from build123d import *

# Parameters (mm, degrees)
F1_DEPTH  = 93
F3_DEPTH  = 25
F4_W      = 3
F4_H      = 15.738895
F4_H_2    = 121.261105
F5_DEPTH  = 15
F6_DEPTH  = 15
F7_DEPTH  = 15
F8_DEPTH  = 15
F9_DEPTH  = 15
F10_DEPTH = 15
F11_DEPTH = 15
F4_H_3    = 121.394625
F12_DEPTH = 15
F13_DEPTH = 15
F14_DEPTH = 15
F15_DEPTH = 15
F16_DEPTH = 15
F17_DEPTH = 15
F18_DEPTH = 15
F19_DEPTH = 15
F20_W     = 23
F20_H     = 10
F21_DEPTH = 0.2
F22_R     = 2.5
F23_DEPTH = 2
F24_DEPTH = 2


with BuildPart() as f1:
    # F0 (on Front) → F1 (new body)
    with BuildSketch(Plane.XZ):
        with BuildLine():
            Line((191.195573, 236.532636), (-173.804427, 236.532636))
            ThreePointArc((-173.804427, 236.532636), (-184.411028, 232.139238), (-188.804427, 221.532636))
            Line((-188.804427, 221.532636), (-188.804427, -78.467364))
            ThreePointArc((-188.804427, -78.467364), (-184.411028, -89.073966), (-173.804427, -93.467364))
            Line((-173.804427, -93.467364), (191.195573, -93.467364))
            Line((191.195573, -93.467364), (191.195573, 236.532636))
        make_face()
        with BuildLine():
            ThreePointArc((-181.804427, 221.532636), (-179.461281, 227.18949), (-173.804427, 229.532636))
            Line((-173.804427, 229.532636), (184.195573, 229.532636))
            Line((184.195573, 229.532636), (184.195573, -86.467364))
            Line((184.195573, -86.467364), (-173.804427, -86.467364))
            ThreePointArc((-173.804427, -86.467364), (-179.461281, -84.124218), (-181.804427, -78.467364))
            Line((-181.804427, -78.467364), (-181.804427, 221.532636))
        make_face(mode=Mode.SUBTRACT)
    extrude(amount=F1_DEPTH)

    # F2 (on face) → F3 (cut)
    with BuildSketch(Plane.YZ.offset(191.195573)):
        Polygon((-6, 128.456), (-6, 226.532636), (-93, 226.532636), (-93, 68.456), (-48, 68.456), (-48, 128.456), align=None)
    extrude(amount=-F3_DEPTH, mode=Mode.SUBTRACT)

    # F4 (on face) → F5 (cut)
    with BuildSketch(Plane(origin=(-188.804427, 0, 0), x_dir=(0, -1, 0), z_dir=(-1, 0, 0))):
        with Locations((88.5, -86.336811)):
            Rectangle(F4_W, F4_H)
        with Locations((88.5, -17.836812)):
            Rectangle(F4_W, F4_H_2)
    extrude(amount=-F5_DEPTH, mode=Mode.SUBTRACT)

    # F4 (on face) → F6 (cut)
    with BuildSketch(Plane(origin=(-188.804427, 0, 0), x_dir=(0, -1, 0), z_dir=(-1, 0, 0))):
        with Locations((82.5, -17.836812)):
            Rectangle(F4_W, F4_H_2)
        with Locations((82.5, -86.336811)):
            Rectangle(F4_W, F4_H)
    extrude(amount=-F6_DEPTH, mode=Mode.SUBTRACT)

    # F4 (on face) → F7 (cut)
    with BuildSketch(Plane(origin=(-188.804427, 0, 0), x_dir=(0, -1, 0), z_dir=(-1, 0, 0))):
        with Locations((76.5, -17.836812)):
            Rectangle(F4_W, F4_H_2)
        with Locations((76.5, -86.336811)):
            Rectangle(F4_W, F4_H)
    extrude(amount=-F7_DEPTH, mode=Mode.SUBTRACT)

    # F4 (on face) → F8 (cut)
    with BuildSketch(Plane(origin=(-188.804427, 0, 0), x_dir=(0, -1, 0), z_dir=(-1, 0, 0))):
        with Locations((70.5, -17.836812)):
            Rectangle(F4_W, F4_H_2)
        with Locations((70.5, -86.336811)):
            Rectangle(F4_W, F4_H)
    extrude(amount=-F8_DEPTH, mode=Mode.SUBTRACT)

    # F4 (on face) → F9 (cut)
    with BuildSketch(Plane(origin=(-188.804427, 0, 0), x_dir=(0, -1, 0), z_dir=(-1, 0, 0))):
        with Locations((64.5, -17.836812)):
            Rectangle(F4_W, F4_H_2)
        with Locations((64.5, -86.336811)):
            Rectangle(F4_W, F4_H)
    extrude(amount=-F9_DEPTH, mode=Mode.SUBTRACT)

    # F4 (on face) → F10 (cut)
    with BuildSketch(Plane(origin=(-188.804427, 0, 0), x_dir=(0, -1, 0), z_dir=(-1, 0, 0))):
        with Locations((58.5, -86.336811)):
            Rectangle(F4_W, F4_H)
        with Locations((58.5, -17.836812)):
            Rectangle(F4_W, F4_H_2)
    extrude(amount=-F10_DEPTH, mode=Mode.SUBTRACT)

    # F4 (on face) → F11 (cut)
    with BuildSketch(Plane(origin=(-188.804427, 0, 0), x_dir=(0, -1, 0), z_dir=(-1, 0, 0))):
        with Locations((52.5, -17.836812)):
            Rectangle(F4_W, F4_H_2)
        with Locations((52.5, -86.336811)):
            Rectangle(F4_W, F4_H)
    extrude(amount=-F11_DEPTH, mode=Mode.SUBTRACT)

    # F4 (on face) → F12 (cut)
    with BuildSketch(Plane(origin=(-188.804427, 0, 0), x_dir=(0, -1, 0), z_dir=(-1, 0, 0))):
        with Locations((46.5, -86.336811)):
            Rectangle(F4_W, F4_H)
        with Locations((46.5, -17.770052)):
            Rectangle(F4_W, F4_H_3)
    extrude(amount=-F12_DEPTH, mode=Mode.SUBTRACT)

    # F4 (on face) → F13 (cut)
    with BuildSketch(Plane(origin=(-188.804427, 0, 0), x_dir=(0, -1, 0), z_dir=(-1, 0, 0))):
        with Locations((40.5, -17.770052)):
            Rectangle(F4_W, F4_H_3)
        with Locations((40.5, -86.336811)):
            Rectangle(F4_W, F4_H)
    extrude(amount=-F13_DEPTH, mode=Mode.SUBTRACT)

    # F4 (on face) → F14 (cut)
    with BuildSketch(Plane(origin=(-188.804427, 0, 0), x_dir=(0, -1, 0), z_dir=(-1, 0, 0))):
        with Locations((40.5, -17.770052)):
            Rectangle(F4_W, F4_H_3)
        with Locations((40.5, -86.336811)):
            Rectangle(F4_W, F4_H)
    extrude(amount=-F14_DEPTH, mode=Mode.SUBTRACT)

    # F4 (on face) → F15 (cut)
    with BuildSketch(Plane(origin=(-188.804427, 0, 0), x_dir=(0, -1, 0), z_dir=(-1, 0, 0))):
        with Locations((34.5, -17.770052)):
            Rectangle(F4_W, F4_H_3)
        with Locations((34.5, -86.336811)):
            Rectangle(F4_W, F4_H)
    extrude(amount=-F15_DEPTH, mode=Mode.SUBTRACT)

    # F4 (on face) → F16 (cut)
    with BuildSketch(Plane(origin=(-188.804427, 0, 0), x_dir=(0, -1, 0), z_dir=(-1, 0, 0))):
        with Locations((28.5, -17.770052)):
            Rectangle(F4_W, F4_H_3)
        with Locations((28.5, -86.336811)):
            Rectangle(F4_W, F4_H)
    extrude(amount=-F16_DEPTH, mode=Mode.SUBTRACT)

    # F4 (on face) → F17 (cut)
    with BuildSketch(Plane(origin=(-188.804427, 0, 0), x_dir=(0, -1, 0), z_dir=(-1, 0, 0))):
        with Locations((22.5, -17.770052)):
            Rectangle(F4_W, F4_H_3)
        with Locations((22.5, -86.336811)):
            Rectangle(F4_W, F4_H)
    extrude(amount=-F17_DEPTH, mode=Mode.SUBTRACT)

    # F4 (on face) → F18 (cut)
    with BuildSketch(Plane(origin=(-188.804427, 0, 0), x_dir=(0, -1, 0), z_dir=(-1, 0, 0))):
        with Locations((16.5, -17.770052)):
            Rectangle(F4_W, F4_H_3)
        with Locations((16.5, -86.336811)):
            Rectangle(F4_W, F4_H)
    extrude(amount=-F18_DEPTH, mode=Mode.SUBTRACT)

    # F4 (on face) → F19 (cut)
    with BuildSketch(Plane(origin=(-188.804427, 0, 0), x_dir=(0, -1, 0), z_dir=(-1, 0, 0))):
        with Locations((10.5, -17.770052)):
            Rectangle(F4_W, F4_H_3)
        with Locations((10.5, -86.336811)):
            Rectangle(F4_W, F4_H)
    extrude(amount=-F19_DEPTH, mode=Mode.SUBTRACT)

    # F20 (on face) → F21 (join)
    with BuildSketch(Plane(origin=(-188.804427, 0, 0), x_dir=(0, -1, 0), z_dir=(-1, 0, 0))):
        with Locations((71.5, 64.793741)):
            Rectangle(F20_W, F20_H)
    extrude(amount=F21_DEPTH)

    # F22 (on face) → F23 (cut)
    with BuildSketch(Plane(origin=(-188.804427, 0, 0), x_dir=(0, -1, 0), z_dir=(-1, 0, 0))):
        with Locations((40, 56.793741)):
            Circle(F22_R)
    extrude(amount=-F23_DEPTH, mode=Mode.SUBTRACT)

    # F22 (on face) → F24 (cut)
    with BuildSketch(Plane(origin=(-188.804427, 0, 0), x_dir=(0, -1, 0), z_dir=(-1, 0, 0))):
        with Locations((40, 72.293741)):
            Circle(F22_R)
    extrude(amount=-F24_DEPTH, mode=Mode.SUBTRACT)


solid = f1.part
Design review of the part built by this model. Coordinates are the model's own, in mm. A direction names the side the tool comes from. Give positions to 0.01 mm unless a question says otherwise; leave off trailing zeros. Write each loop counter-clockwise with the first axis right and the second up, starting at its lowest first coordinate (ties: lowest second). Pieces come first, ordered by that corner, then holes. Notation, with made-up numbers: M 85.25,-27 L 129.25,-27 A18 cw 129.25,-3 Z; hole C -31.75,72.5 d3. An arc over 180 degrees is marked long. Answer as a JSON object with one key per item and string values. Group by question number.
1) We need section B-B (x = 159.5). Give the boundary of the cut face in (y, z), and give its area (3 significant figures).
2) Clearance check with flat-ended pins moving along their axes: pin 1 Ø2.5 at (x, y) = (-184, -82.5) entering from -Z; pin 2 Ø3 at (y, z) = (-24.5, 196.5) entering from -X; pin 3 Ø1.5 at (y, z) = (-64, 22.5) entering from -X. State where each tip first meets the part, or that it passes through.
3) For line 1 along Z through (x, y) = (147.5, -45); line 2 along X through (y, z) = (-27, 95); line 3 along Z through (x, y) = (-187, -40), list the stretches that pass through material, from the lowest coordinate up.
4) Mouldability with a two-part tool opening along Y and no side actions: class faces 1 (the face through (-183, -93, 72)), 2 (the face through (-185, -24, -26)), 3 (the face through (-184.527, -49.479, -88.957)) as released by +Y, released by -Y, zero draft, split by the parting line, or undercut.
5) Tool access review of faces 4 (the face through (-185, -33, -24)), 5 (the face through (191.196, -36, -4)), 6 (the face through (-179.399, -79.479, -84.186)): name each direction out of +Z, -Z, +X, -X, +Y, -Y from which nothing blocks a thin tool from reaching the whole face with its end or side.
6) We need section A-A (z = 183.5). Give the boundary of the cut face in (x, y), and give its area (3 significant figures).
7) We need section C-C (z = -19). Count the separate pieces of the cut face and the enclosed holes in it, and give its area (3 significant figures).
Answer key:
{
 "1": {"outline": "M -93,-93.47 L 0,-93.47 L 0,-86.47 L -93,-86.47 Z; M -93,229.53 L 0,229.53 L 0,236.53 L -93,236.53 Z", "area": "1,300 mm²"},
 "2": {"pin 1": "stops at z = 42.79", "pin 2": "stops at x = -188.8", "pin 3": "stops at x = 184.2"},
 "3": {"line 1": "z = -93.47 to -86.47, 229.53 to 236.53", "line 2": "x = -188.8 to -181.8, 184.2 to 191.2", "line 3": "z = 42.93 to 54.29, 59.29 to 69.79, 74.79 to 228.67"},
 "4": {"face 1": "released by -Y", "face 2": "undercut", "face 3": "zero draft"},
 "5": {"face 4": "-Z, -X", "face 5": "+Z, -Z, +X, +Y, -Y", "face 6": "+Y, -Y"},
 "6": {"outline": "M -188.8,-93 L -181.8,-93 L -181.8,0 L -188.8,0 Z; M 184.2,-6 L 191.2,-6 L 191.2,0 L 184.2,0 Z", "area": "693 mm²"},
 "7": {"separate pieces": "16", "enclosed holes": "0", "area": "1,010 mm²"}
}
